Autodesk Inventor part; units mm, degrees
ref_plane "YZ Plane" through (0, 0, 0) normal (1, 0, 0) x (0, 1, 0)
ref_plane "XZ Plane" through (0, 0, 0) normal (0, 1, 0) x (-1, 0, 0)
ref_plane "XY Plane" through (0, 0, 0) normal (0, 0, 1) x (1, 0, 0)
sketch "Sketch1" plane through (0, 0, 0) normal (0, 1, 0) x (-1, 0, 0)
  circle A0 centre (0, 0) radius 11
  circle A1 centre (0, 0) radius 20
  dimension "d0" = 22
  dimension "d1" = 40
extrude "Extrusion1" add sketch "Sketch1" along normal blind 7
sketch "Sketch2" plane through (0, 0, 0) normal (1, 0, 0) x (0, 1, 0)
  line L0 (0, 40.32) -> (7.62, 40.32)
  line L1 (7.62, 40.32) -> (7.62, 53.02)
  line L2 (7.62, 53.02) -> (0, 53.02)
  line L3 (0, 53.02) -> (0, 40.32)
  line L4 (0, 40.32) -> (3.81, 40.32)
  line L5 (3.81, 40.32) -> (3.81, 20)
  line L6 (3.81, 20) -> (0, 20)
  line L7 (0, 20) -> (0, 40.32)
  line L8 (-1.524, 0) -> (9.144, 0)
  point P0 (0, 0)
  dimension "d4" = 20.32
  dimension "d5" = 7.62
  dimension "d6" = 20
  dimension "d7" = 3.81
  dimension "d8" = 12.7
revolve "Revolution1" add sketch "Sketch2" angle 360 about axis through (0, -10, 0) along (0, 1, 0)
sketch "Sketch3" plane through (0, 3.81, 0) normal (0, 1, 0) x (1, 0, 0)
  circle A0 centre (0, 0) radius 40.32 construction
  circle A1 centre (0, 0) radius 20 construction
  circle A2 centre (0, 30.16) radius 3.175
  line L0 (0, 30.16) -> (0, 20)
  line L1 (0, 30.16) -> (0, 40.32)
  circle A3 centre (-26.1193, 15.08) radius 3.175
  circle A4 centre (-26.1193, -15.08) radius 3.175
  circle A5 centre (0, -30.16) radius 3.175
  circle A6 centre (26.1193, -15.08) radius 3.175
  circle A7 centre (26.1193, 15.08) radius 3.175
  dimension "d10" = 6.35
  dimension "d13" = 360
extrude "Extrusion2" cut sketch "Sketch3" against normal blind 7
properties part number "OuterBearingHolder"
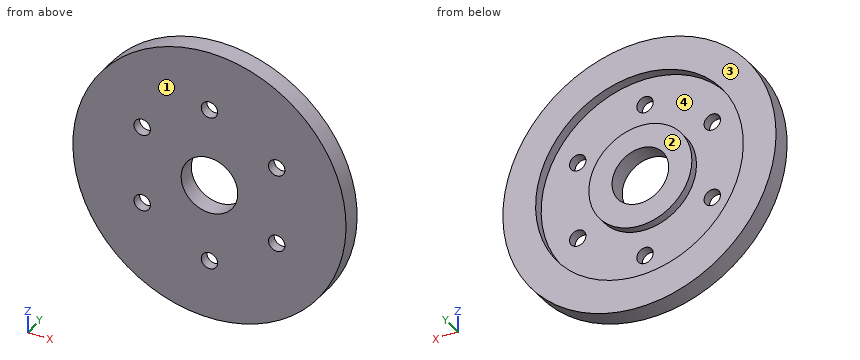
Verification items for the finished model (mm, model axes). Face numbers are marked on the shaded views. A direction names the side the tool comes from. Coordinates: 2 decimals unless noted, no trailing zeros. Order: outer loops, then holes, each group sorted by start corner. A loop starts at its lowest first (then second) coordinate and runs counter-clockwise, first axis right, second up.
Item 1: Material ranges on L1, parallel to Z at x = 28, y = 1.5; L2, parallel to X at y = 1.2, z = -15.08; L3, parallel to Y at x = -16, z = -4.5, recorded low to high.
Filled in:
L1: z = -45.02 to -17.64, -12.52 to 12.52, 17.64 to 45.02
L2: x = -50.83 to -29.29, -22.94 to 22.94, 29.29 to 50.83
L3: y = 0 to 7
Item 2: Section check C-C, the plane x = 5.5. Enter the section's corners in (y, z).
Filled in:
outline: (0, -52.73) - (7.62, -52.73) - (7.62, -39.94) - (3.81, -39.94) - (3.81, -19.23) - (7, -19.23) - (7, -9.53) - (0, -9.53) - close; (0, 9.53) - (7, 9.53) - (7, 19.23) - (3.81, 19.23) - (3.81, 39.94) - (7.62, 39.94) - (7.62, 52.73) - (0, 52.73) - close
Item 3: Section check A-A, the plane z = 0. Enter the section's corners in (x, y), then the cut area to 3 significant figures.
Filled in:
outline: (-53.02, 0) - (-11, 0) - (-11, 7) - (-20, 7) - (-20, 3.81) - (-40.32, 3.81) - (-40.32, 7.62) - (-53.02, 7.62) - close; (11, 0) - (53.02, 0) - (53.02, 7.62) - (40.32, 7.62) - (40.32, 3.81) - (20, 3.81) - (20, 7) - (11, 7) - close
area: 474 mm2
Item 4: Release check for a two-part mould opening along X. For the marked faces 3 and 4 record: +X half, -X half, draft (parallel to the pull), parting line (faces both ways), or undercut.
Filled in:
face 3: draft
face 4: undercut
Item 5: Section check D-D, the plane z = -15.08. Enter the section's corners in (x, y).
Filled in:
outline: (-50.83, 0) - (-29.29, 0) - (-29.29, 3.81) - (-37.39, 3.81) - (-37.39, 7.62) - (-50.83, 7.62) - close; (-22.94, 0) - (22.94, 0) - (22.94, 3.81) - (13.14, 3.81) - (13.14, 7) - (-13.14, 7) - (-13.14, 3.81) - (-22.94, 3.81) - close; (29.29, 0) - (50.83, 0) - (50.83, 7.62) - (37.39, 7.62) - (37.39, 3.81) - (29.29, 3.81) - close
Item 6: Access from +Z, -Z, +X, -X, +Y, -Y to the whole of each face (thin tool, end or side, straight path). Record for the marked faces 1 and 2.
Filled in:
face 1: +Z, -Z, +X, -X, -Y
face 2: +Y
Item 7: Depth check by flat-ended pin: pin 1 (1 mm diameter, centred on x = -6, z = -28, fed in from +Y); pin 2 (4 mm diameter, centred on x = -36, y = 5, fed in from -Z); pin 3 (5.5 mm diameter, centred on x = 26.12, z = -15.08, fed in from +Y); pin 4 (4 mm diameter, centred on x = -40, y = 5, fed in from -Z). Enter the tip coordinate at first touch or a pass-through.
Filled in:
pin 1: stops at y = 3.81
pin 2: stops at z = -40.68
pin 3: passes through
pin 4: stops at z = -36.97
Item 8: Section check B-B, the plane y = 5. Enter the section's corners in (x, z).
Filled in:
outline: circle Ø106.04 at (0, 0); circle Ø40 at (0, 0); hole circle Ø80.64 at (0, 0); hole circle Ø22 at (0, 0)
